Model file for the job. Use its own axes, mm. Face numbers are marked on the shaded views. A direction names the side the tool comes from. Round coordinates to 2 decimals unless told otherwise and drop trailing zeros. Order: outer loops, then holes, each group sorted by start corner. A loop starts at its lowest first (then second) coordinate and runs counter-clockwise, first axis right, second up. Notation, with made-up numbers: (-2.75, 64) - (36.25, 64) arc R27 ccw to (36.25, 102) - close; hole circle Ø7 at (58.5, 62.25). An arc over 180 degrees is marked (long way). Answer as CSV lines item,"result". Start each with the question number.
1. 3-axis set-ups, long thin cutter, end or side, ignore diameter. For the marked faces 4 and 5: which of +Z, -Z, +X, -X, +Y, -Y reach the whole face in a straight line?
2. Band-saw the part on A-A on z = -6.75. List the corners of the cut face in (x, y), then the cut area to 3 significant figures.
3. Band-saw the part on B-B on y = 9.25. List the corners of the cut face in (x, z).
4. Wall check: line 1 along X through (y, z) = (8.25, -2.5); line 2 along X through (y, z) = (6.5, -15); line 3 along Y through (x, z) = (7, -15.5). Give the ranges that are in metal, low to high. Write a range as [from, to].
5. Band-saw the part on C-C on x = 51.5. List the corners of the cut face in (y, z), then the cut area to 3 significant figures.
6. Pull direction X, two halves, no side cores. Call the marked faces 1, 2 and 3: released by +X, released by -X, zero draft, split by the parting line, or undercut.
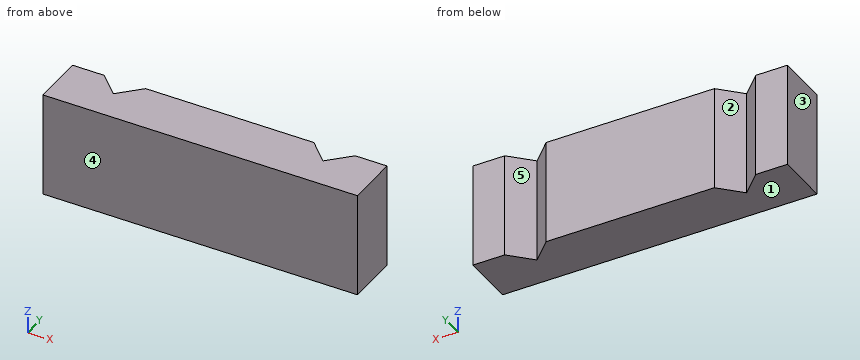
```python
from build123d import *

# Parameters (mm, degrees)
SKETCH1_W           = 60
SKETCH1_H           = 20
BOSS_EXTRUDE1_DEPTH = 10
CUT_EXTRUDE1_DEPTH  = 65.031242374


with BuildPart() as part:
    # Sketch1 → Boss-Extrude1 (new body)
    with BuildSketch(Plane(origin=(0, 0, 0), x_dir=(1, 0, 0), z_dir=(0, 1, 0))):
        with Locations((30, 10)):
            Rectangle(SKETCH1_W, SKETCH1_H)
    extrude(amount=BOSS_EXTRUDE1_DEPTH)

    # Sketch2 → Cut-Extrude1 (cut, through all)
    with BuildSketch(Plane.XY):
        Polygon((13.94522636, 10), (6.05477364, 10), (10, 6.05477364), align=None)
        Polygon((46.05477364, 10), (50, 6.05477364), (53.94522636, 10), align=None)
    extrude(amount=-CUT_EXTRUDE1_DEPTH, mode=Mode.SUBTRACT)


solid = part.part
```
Reply:
1,face 4,"+Z, -Z, +X, -X, -Y"
1,face 5,"+Z, -Z, +Y"
2,outline,"(0, 0) - (60, 0) - (60, 10) - (53.95, 10) - (50, 6.05) - (46.05, 10) - (13.95, 10) - (10, 6.05) - (6.05, 10) - (0, 10) - close"
2,area,"569 mm2"
3,outline,"(0, -20) - (6.8, -20) - (6.8, 0) - (0, 0) - close; (13.2, -20) - (46.8, -20) - (46.8, 0) - (13.2, 0) - close; (53.2, -20) - (60, -20) - (60, 0) - (53.2, 0) - close"
4,line 1,"x = [0, 7.8], [12.2, 47.8], [52.2, 60]"
4,line 2,"x = [0, 9.55], [10.45, 49.55], [50.45, 60]"
4,line 3,"y = [0, 9.05]"
5,outline,"(0, -20) - (7.55, -20) - (7.55, 0) - (0, 0) - close"
5,area,"151 mm2"
6,face 1,"zero draft"
6,face 2,"undercut"
6,face 3,"released by -X"
